CAD build for the part. Positions are in the model's coordinates, mm. Give positions to 0.01 mm unless a question says otherwise; leave off trailing zeros.
from build123d import *

# Parameters (mm, degrees)
BOSS_EXTRUDE1_DEPTH         = 1.6
HOLE_WIZARD_2_2_2_2_1_D     = 2.2
HOLE_WIZARD_2_2_2_2_1_DEPTH = 2
SKETCH12_R                  = 1.5
CUT_EXTRUDE1_DEPTH          = 2.6
HOLE_WIZARD_2_2_2_2_2_D     = 2.2
HOLE_WIZARD_2_2_2_2_2_DEPTH = 1.6


with BuildPart() as part:
    # Sketch1 → Boss-Extrude1 (new body)
    with BuildSketch(Plane(origin=(0, 0, 0), x_dir=(1, 0, 0), z_dir=(0, 1, 0))):
        Polygon((-35.644384454, 8.907074992), (-28.844384454, 8.907074992), (-28.844384454, 15.707074992), (52.055615546, 15.707074992), (52.055615546, 8.907074992), (60.355615546, 8.907074992), (60.355615546, -73.492925008), (53.555615546, -73.492925008), (53.555615546, -80.292925008), (-27.344384454, -80.292925008), (-27.344384454, -73.492925008), (-35.644384454, -73.492925008), align=None)
    extrude(amount=BOSS_EXTRUDE1_DEPTH)

    # Ø2.2 (2.2) 直径の穴1
    with Locations(Plane(origin=(0, 1.6, 0), x_dir=(1, 0, 0), z_dir=(0, 1, 0))):
        with Locations((57.855615546, -32.292925008), (-33.144384454, -32.292925008), (41.855615546, -78.192925008), (41.855615546, 13.607074992), (-17.144384454, 13.607074992), (-17.144384454, -78.192925008)):
            Hole(HOLE_WIZARD_2_2_2_2_1_D / 2, depth=HOLE_WIZARD_2_2_2_2_1_DEPTH)

    # Sketch12 → Cut-Extrude1 (cut, through all)
    with BuildSketch(Plane(origin=(0, 1.6, 0), x_dir=(1, 0, 0), z_dir=(0, 1, 0))):
        with Locations((53.555615546, 8.907074992)):
            Circle(SKETCH12_R)
        with Locations((-28.844384454, -73.492925008)):
            Circle(SKETCH12_R)
    extrude(amount=-CUT_EXTRUDE1_DEPTH, mode=Mode.SUBTRACT)

    # Ø2.2 (2.2) 直径の穴2
    with Locations(Plane(origin=(0, 1.6, 0), x_dir=(1, 0, 0), z_dir=(0, 1, 0))):
        with Locations((-33.344384454, 2.207074992), (-33.344384454, -66.792925008), (58.055615546, -66.792925008), (58.055615546, 2.207074992)):
            Hole(HOLE_WIZARD_2_2_2_2_2_D / 2, depth=HOLE_WIZARD_2_2_2_2_2_DEPTH)


solid = part.part
1. Saw through at A-A on y = 1. State how many separate pieces and enclosed holes the cut face has, plus the area to 3 significant figures.
2. Wall check: line 1 (Z direction, x = 42, y = 1.2); line 2 (X direction, y = 0.25, z = -12); line 3 (Z direction, x = -28, y = 0.45). Give the ranges that are in metal, low to high.
3. Mould opens along Z. For faces 1 (the flat face through (13, 0, 32)), 2 (the cylindrical face through (-16.3, 0.8, -12.9)) say: released by +Z, released by -Z, zero draft, split by the parting line, or undercut.
4. Pin check, flat tips, straight feed: P1, Ø0.5, axis at y = 0.5, z = -12.5, coming from the -X side; P2, Ø0.5, axis at y = 1, z = 77, coming from the -X side; P3, Ø0.8, axis at y = 1, z = -11, coming from the +X side; P4, Ø1.8, axis at x = 58.06, z = 66.79, coming from the +Y side. Stop position of each tip, or through.
Reported:
1. separate pieces: 1
1. enclosed holes: 10
1. area: 8,970 mm2
2. line 1: z = -15.71 to -14.7, -12.52 to 77.1, 79.28 to 80.29
2. line 2: x = -28.84 to 52.06
2. line 3: z = -15.71 to 72.25
3. face 1: zero draft
3. face 2: undercut
4. P1: stops at x = -28.84
4. P2: stops at x = -27.34
4. P3: stops at x = 52.06
4. P4: passes through
